```python
from build123d import *

# Parameters (mm, degrees)
F1_DEPTH = 10
F2_F1_R  = 8.2083261121
F2_F2_R  = 8.2083261121


with BuildPart() as f1:
    # F0 (on Right) → F1 (new body, symmetric)
    with BuildSketch(Plane.YZ):
        Polygon((-255.1260930291, 127.6137977839), (-296.4929085316, 127.6137977839), (-296.4929085316, 0), (-262.0377242565, 0), (-241.1511396352, 11.6772135656), (-177.6259690523, 47.1926890314), (-130.9504058889, 47.1926890314), (-86.4829342095, 47.1926890314), (-44.2343052483, 47.1926890314), (6.9967018189, 47.1926890314), (303.5070914684, 47.1926890314), (303.5070914684, 127.6137977839), (-89.1410559416, 127.6137977839), (-137.561365962, 107.9020351171), (-232.3477119207, 107.9020351171), align=None)
        Polygon((-241.1511396352, 11.6772135656), (-262.0377242565, 0), (-77.4150533853, 0), (6.9967018189, 47.1926890314), (-44.2343052483, 47.1926890314), (-44.2343052483, 34.5198116153), (-85.0919854182, 11.6772135656), (-150.0081047923, 11.6772135656), (-194.4755764717, 11.6772135656), align=None)
        Polygon((-130.9504058889, 47.1926890314), (-194.4755764717, 11.6772135656), (-150.0081047923, 11.6772135656), (-86.4829342095, 47.1926890314), align=None)
    extrude(amount=F1_DEPTH, both=True)

    # F2: fillet of radius 8.2083261121 on 12 edges, made by hand

    # F2_f1
    f2_f1_edges = [f1.edges().sort_by_distance(p)[0] for p in [
        (0, -150.0081047923, 11.6772135656),
        (0, -194.4755764717, 11.6772135656),
        (0, -85.0919854182, 11.6772135656),
        (0, -44.2343052483, 34.5198116153),
    ]]
    fillet(f2_f1_edges, radius=F2_F1_R)

    # F2_f2
    f2_f2_edges = [f1.edges().sort_by_distance(p)[0] for p in [
        (10, -161.7795821345, 29.9567990284),
        (-10, -161.7795821345, 29.9567990284),
        (-10, -104.4970100413, 37.1214296806),
        (10, -104.4970100413, 37.1214296806),
        (10, -126.4486219722, 17.8158787517),
        (-10, -126.4486219722, 17.8158787517),
        (-10, -194.5446792073, 11.9424218254),
        (10, -194.5446792073, 11.9424218254),
    ]]
    fillet(f2_f2_edges, radius=F2_F2_R)


solid = f1.part
```
Could you check a few things on this model? Use its own coordinates, in mm. A direction names the side the tool comes from. Coordinates: 2 decimals unless noted, no trailing zeros. Loops run counter-clockwise (first coordinate to the right, second up) from the corner with the lowest first, then second, coordinate; pieces in that order, holes last. Notation, with made-up numbers: M 8,19.5 L 47,19.5 A21 ccw 47,42.5 Z; hole C -38.5,-8.5 d4. An arc over 180 degrees is marked long. Put each result on its own line as item: value. Start each with the question number.
(1) Will these pins go through, and if not, where does the flat tip stop? P1, Ø4, axis at x = 0.5, y = -224.5, coming from the +Z side; P2, Ø6, axis at x = 3, y = 216.5, coming from the -Z side; P3, Ø6, axis at x = 4, y = -71.5, coming from the -Z side; P4, Ø10, axis at x = 4, y = -152.5, coming from the -Z side.
(2) Thinking about a two-plate mould opening in Y: for faces 5 (the face through (0, -184, 107.902)), 6 (the face through (0.14, -35.8, 23.266)), 7 (the face through (0, 153, 47.193)), which applies, pulls with the +Y half, pulls with the -Y half, needs draft (parallel to the pull), parting line crosses it, or undercut?
(3) Suppose I cut it at B-B on x = -5. Please give me the cut outline in (y, z), then the cut area to 3 significant figures.
(4) Suppose I cut it at C-C on y = 170. Please give me the cut outline in (x, z).
(5) Suppose I cut it at A-A on y = -223.5. Please give me the cut outline in (x, z), then the cut area to 3 significant figures.
(6) Suppose I cut it at D-D on y = -22. Please give me the cut outline in (x, z).
(7) For faces 1 (the face through (7.659, -64.87, 20.155)), 2 (the face through (0.025, -161.348, 30.198)), 3 (the face through (0.14, -243.58, 117.62)), 4 (the face through (-7.53, -64.93, 20.27)), which set-ups out of +Z, -Z, +X, -X, +Y, -Y let a thin tool reach every point of the face, with its end or its side?
(8) I need wall thicknesses on line 1 (Y direction, x = 7.5, z = 22); line 2 (Z direction, x = 3.5, y = -116.5); line 3 (Z direction, x = -3.75, y = 89). Which ranges of each line are inside material? Lowest first, please. Write a range as from..to.
Solutions:
1. P1: stops at z = 107.9
1. P2: stops at z = 47.19
1. P3: stops at z = 1.63
1. P4: stops at z = 0
2. face 5: undercut
2. face 6: pulls with the +Y half
2. face 7: needs draft
3. outline: M -296.49,0 L -77.42,0 L 7,47.19 L 303.51,47.19 L 303.51,127.61 L -89.14,127.61 L -137.56,107.9 L -232.35,107.9 L -255.13,127.61 L -296.49,127.61 Z; hole M -242.32,11.02 L -196.61,11.02 A8.86 ccw -192.29,12.15 L -129.61,47.19 L -177.63,47.19 Z; hole M -122.83,27.62 A8.86 ccw -118.51,11.02 L -87.23,11.02 A8.86 ccw -82.91,12.15 L -48.12,31.6 A8.86 ccw -43.58,39.33 L -43.58,47.19 L -87.82,47.19 Z
3. area: 54,200 mm2
4. outline: M -10,47.19 L 10,47.19 L 10,127.61 L -10,127.61 Z
5. outline: M -10,0 L 10,0 L 10,3.47 A8.21 ccw 1.79,11.68 L -1.79,11.68 A8.21 ccw -10,3.47 Z; M -10,21.55 L 10,21.55 L 10,107.9 L -10,107.9 Z
5. area: 1,930 mm2
6. outline: M -10,30.98 L 10,30.98 L 10,127.61 L -10,127.61 Z
7. face 1: +X
7. face 2: +X, -X
7. face 3: +Z, +X, -X
7. face 4: -X
8. line 1: y = -296.49..-222.69, -171.28..-128.81, -61.89..-38.06
8. line 2: z = 0..11.5, 30.62..116.48
8. line 3: z = 47.19..127.61
